Input: part model. Units: mm. Frame: model coordinates. A direction names the side the tool comes from. Coordinates: 2 decimals unless noted, no trailing zeros. Loops run counter-clockwise (first coordinate to the right, second up) from the corner with the lowest first, then second, coordinate; pieces in that order, holes last.
Item 1: Section C-C on z = 1. Give the number of separate pieces and of enclosed holes in the cut face, and give its area (3 significant figures).
Item 2: Section A-A on z = 113. Return loops of the section in (x, y).
Item 3: Reachability of faces 4 (the cylindrical face through (13.086, 15.703, 37.874)), 5 (the cylindrical face through (251.818, 100.714, 47.439)), 6 (the cylindrical face through (209.86, -93.2, -12.24)) from +Z, -Z, +X, -X, +Y, -Y: full face, straight path, thin tool, end or side. Return the list, or none.
Item 4: Ray query, line 1 along Y through (x, z) = (244.5, -56.5); line 2 along Y through (x, z) = (38.5, -2); line 3 along Y through (x, z) = (27, 23). Return the intervals inside material, ascending.
Item 5: Contact query for flat-ended pins moving along their axis: P1, Ø4, axis at y = -60.5, z = -50, coming from the -X side; P2, Ø15, axis at y = -56.5, z = -97.86, coming from the +X side; P3, Ø6, axis at x = 230, y = -85.5, coming from the -Z side; P4, Ø6, axis at x = 128.5, y = 33.5, coming from the -Z side. Output: stop coordinate, or through.
Item 6: Pull-direction query (X, two-part tool) for faces 1 (the conical face through (1.594, 25.1, -32.735)), 2 (the cylindrical face through (251.82, -62.28, 105.4)), 3 (the flat face through (0, -10.6, 29.4)); classes: released by +X, released by -X, zero draft, split by the parting line, or undercut.
```python
from build123d import *

# Parameters (mm, degrees)
SKETCH_3_R           = 9.5
CUT_EXTRUDE_1_DEPTH  = 321.526909947
SKETCH_4_R           = 9.5
CUT_EXTRUDE_2_DEPTH  = 321.526909947
SKETCH_5_R           = 9.5
CUT_EXTRUDE_3_DEPTH  = 321.526909947
SKETCH_6_R           = 9.5
CUT_EXTRUDE_4_DEPTH  = 321.526909947
SKETCH_7_R           = 9.5
CUT_EXTRUDE_5_DEPTH  = 321.526909947
SKETCH_8_R           = 9.5
CUT_EXTRUDE_6_DEPTH  = 321.526909947
SKETCH_9_R           = 9.5
CUT_EXTRUDE_7_DEPTH  = 321.526909947
SKETCH_10_R          = 9.5
CUT_EXTRUDE_8_DEPTH  = 321.526909947
SKETCH_11_R          = 9.5
CUT_EXTRUDE_9_DEPTH  = 321.526909947
SKETCH_12_R          = 9.5
CUT_EXTRUDE_10_DEPTH = 321.526909947
SKETCH_13_R          = 9.5
CUT_EXTRUDE_11_DEPTH = 321.526909947
SKETCH_14_R          = 9.5
CUT_EXTRUDE_12_DEPTH = 321.526909947


with BuildPart() as part:
    # Эскиз1 → Повернуть1 (revolve)
    with BuildSketch(Plane.XY, mode=Mode.PRIVATE) as revolve_1_sk:
        Polygon((0, 0), (265, 0), (265, 127.5), (239, 127.5), (239, 100), (239, 95), (220, 95), (220, 94), (200, 94), (144, 65.5), (70, 65.5), (25, 41), (1.5, 41), (3, 45), (0, 45), align=None)
    revolve(revolve_1_sk.sketch.rotate(Axis((0, 0, 0), (1, 0, 0)), 90), axis=Axis((0, 0, 0), (1, 0, 0)))

    # Эскиз2 → Вырез-Повернуть1 (revolve, cut)
    with BuildSketch(Plane.XY, mode=Mode.PRIVATE) as cut_revolve_1_sk:
        with BuildLine():
            Line((0, 0), (140, 0))
            Line((140, 0), (140, 52.583909796))
            Line((140, 52.583909796), (124.820646354, 52.583909796))
            ThreePointArc((124.820646354, 52.583909796), (118.294984956, 52.093441156), (111.880765, 50.796291))
            Line((111.880765, 50.796291), (38, 31))
            Line((38, 31), (0, 31))
            Line((0, 31), (0, 0))
        make_face()
    revolve(cut_revolve_1_sk.sketch.rotate(Axis((0, 0, 0), (1, 0, 0)), 90), axis=Axis((0, 0, 0), (1, 0, 0)), mode=Mode.SUBTRACT)

    # Эскиз3 → Вырез-Вытянуть1 (cut, through all)
    with BuildSketch(Plane(origin=(0, 0, 0), x_dir=(0, 0, -1), z_dir=(1, 0, 0))):
        with Locations((0, 113)):
            Circle(SKETCH_3_R)
    extrude(amount=CUT_EXTRUDE_1_DEPTH, mode=Mode.SUBTRACT)

    # Эскиз4 → Вырез-Вытянуть2 (cut, through all)
    with BuildSketch(Plane(origin=(0, 0, 0), x_dir=(0, 0, -1), z_dir=(1, 0, 0))):
        with Locations((-56.5, 97.860870628)):
            Circle(SKETCH_4_R)
    extrude(amount=CUT_EXTRUDE_2_DEPTH, mode=Mode.SUBTRACT)

    # Эскиз5 → Вырез-Вытянуть3 (cut, through all)
    with BuildSketch(Plane(origin=(0, 0, 0), x_dir=(0, 0, -1), z_dir=(1, 0, 0))):
        with Locations((-97.860870628, 56.5)):
            Circle(SKETCH_5_R)
    extrude(amount=CUT_EXTRUDE_3_DEPTH, mode=Mode.SUBTRACT)

    # Эскиз6 → Вырез-Вытянуть4 (cut, through all)
    with BuildSketch(Plane(origin=(0, 0, 0), x_dir=(0, 0, -1), z_dir=(1, 0, 0))):
        with Locations((-113, 0)):
            Circle(SKETCH_6_R)
    extrude(amount=CUT_EXTRUDE_4_DEPTH, mode=Mode.SUBTRACT)

    # Эскиз7 → Вырез-Вытянуть5 (cut, through all)
    with BuildSketch(Plane(origin=(0, 0, 0), x_dir=(0, 0, -1), z_dir=(1, 0, 0))):
        with Locations((-97.860870628, -56.5)):
            Circle(SKETCH_7_R)
    extrude(amount=CUT_EXTRUDE_5_DEPTH, mode=Mode.SUBTRACT)

    # Эскиз8 → Вырез-Вытянуть6 (cut, through all)
    with BuildSketch(Plane(origin=(0, 0, 0), x_dir=(0, 0, -1), z_dir=(1, 0, 0))):
        with Locations((-56.5, -97.860870628)):
            Circle(SKETCH_8_R)
    extrude(amount=CUT_EXTRUDE_6_DEPTH, mode=Mode.SUBTRACT)

    # Эскиз9 → Вырез-Вытянуть7 (cut, through all)
    with BuildSketch(Plane(origin=(0, 0, 0), x_dir=(0, 0, -1), z_dir=(1, 0, 0))):
        with Locations((0, -113)):
            Circle(SKETCH_9_R)
    extrude(amount=CUT_EXTRUDE_7_DEPTH, mode=Mode.SUBTRACT)

    # Эскиз10 → Вырез-Вытянуть8 (cut, through all)
    with BuildSketch(Plane(origin=(0, 0, 0), x_dir=(0, 0, -1), z_dir=(1, 0, 0))):
        with Locations((56.5, -97.860870628)):
            Circle(SKETCH_10_R)
    extrude(amount=CUT_EXTRUDE_8_DEPTH, mode=Mode.SUBTRACT)

    # Эскиз11 → Вырез-Вытянуть9 (cut, through all)
    with BuildSketch(Plane(origin=(0, 0, 0), x_dir=(0, 0, -1), z_dir=(1, 0, 0))):
        with Locations((97.860870628, -56.5)):
            Circle(SKETCH_11_R)
    extrude(amount=CUT_EXTRUDE_9_DEPTH, mode=Mode.SUBTRACT)

    # Эскиз12 → Вырез-Вытянуть10 (cut, through all)
    with BuildSketch(Plane(origin=(0, 0, 0), x_dir=(0, 0, -1), z_dir=(1, 0, 0))):
        with Locations((113, 0)):
            Circle(SKETCH_12_R)
    extrude(amount=CUT_EXTRUDE_10_DEPTH, mode=Mode.SUBTRACT)

    # Эскиз13 → Вырез-Вытянуть11 (cut, through all)
    with BuildSketch(Plane(origin=(0, 0, 0), x_dir=(0, 0, -1), z_dir=(1, 0, 0))):
        with Locations((97.860870628, 56.5)):
            Circle(SKETCH_13_R)
    extrude(amount=CUT_EXTRUDE_11_DEPTH, mode=Mode.SUBTRACT)

    # Эскиз14 → Вырез-Вытянуть12 (cut, through all)
    with BuildSketch(Plane(origin=(0, 0, 0), x_dir=(0, 0, -1), z_dir=(1, 0, 0))):
        with Locations((56.5, 97.860870628)):
            Circle(SKETCH_14_R)
    extrude(amount=CUT_EXTRUDE_12_DEPTH, mode=Mode.SUBTRACT)


solid = part.part
```
Results found:
1. separate pieces: 3
1. enclosed holes: 0
1. area: 27,200 mm2
2. outline: (239, -59.05) - (265, -59.05) - (265, -9.5) - (239, -9.5) - close; (239, 9.5) - (265, 9.5) - (265, 59.05) - (239, 59.05) - close
3. face 4: none
3. face 5: +X, -X
3. face 6: -X
4. line 1: y = -114.3 to -107.36, -88.36 to 88.36, 107.36 to 114.3
4. line 2: y = -48.31 to -31.07, 31.07 to 48.31
4. line 3: y = -35.25 to -20.78, 20.78 to 35.25
5. P1: stops at x = 165.59
5. P2: passes through
5. P3: stops at z = -47.1
5. P4: stops at z = -57.97
6. face 1: undercut
6. face 2: zero draft
6. face 3: released by -X
